```python
from build123d import *

# Parameters (mm, degrees)
SKETCH_1_W          = 56.5
SKETCH_1_H          = 65.5
EXTRUDE_1_DEPTH     = 1.5
SKETCH_2_W          = 59
SKETCH_2_H          = 68
SKETCH_2_W_2        = 56.5
SKETCH_2_H_2        = 65.5
EXTRUDE_2_DEPTH     = 3
FILLET_1_R          = 0.3
SKETCH_4_W          = 25
SKETCH_4_H          = 5
SKETCH_4_W_2        = 30.699386717
SKETCH_4_H_2        = 8.5
SKETCH_4_W_3        = 20
SKETCH_4_H_3        = 30
CUT_EXTRUDE_1_DEPTH = 1
SKETCH_5_W          = 17.035074377
SKETCH_5_H          = 1.25
CUT_EXTRUDE_2_DEPTH = 1.5


with BuildPart() as part:
    # 草图1 → 凸台-拉伸1 (new body)
    with BuildSketch(Plane.XY):
        Rectangle(SKETCH_1_W, SKETCH_1_H)
    extrude(amount=EXTRUDE_1_DEPTH)

    # 草图2 → 凸台-拉伸2 (add)
    with BuildSketch(Plane.XY.offset(1.5)):
        Rectangle(SKETCH_2_W, SKETCH_2_H)
        Rectangle(SKETCH_2_W_2, SKETCH_2_H_2, mode=Mode.SUBTRACT)
    extrude(amount=-EXTRUDE_2_DEPTH)

    # 圆角1
    fillet_1_edges = [part.edges().sort_by_distance(p)[0] for p in [
        (29.5, 34, 0),
        (29.5, -34, 0),
        (-29.5, -34, 0),
        (-29.5, 34, 0),
        (29.5, 0, 1.5),
        (0, 34, 1.5),
        (-29.5, 0, 1.5),
        (0, -34, 1.5),
    ]]
    fillet(fillet_1_edges, radius=FILLET_1_R)

    # 草图4 → 切除-拉伸1 (cut)
    with BuildSketch(Plane(origin=(0, 0, 0), x_dir=(-1, 0, 0), z_dir=(0, 0, -1))):
        with Locations((7.75, 13.75)):
            Rectangle(SKETCH_4_W, SKETCH_4_H)
        with Locations((5.900306641, 5.5)):
            Rectangle(SKETCH_4_W_2, SKETCH_4_H_2)
        with Locations((11.25, -15.75)):
            Rectangle(SKETCH_4_W_3, SKETCH_4_H_3)
    extrude(amount=-CUT_EXTRUDE_1_DEPTH, mode=Mode.SUBTRACT)

    # 草图5 → 切除-拉伸2 (cut)
    with BuildSketch(Plane(origin=(0, 0, -1.5), x_dir=(-1, 0, 0), z_dir=(0, 0, -1))):
        with Locations((-15.836199448, 33.375)):
            Rectangle(SKETCH_5_W, SKETCH_5_H)
    extrude(amount=-CUT_EXTRUDE_2_DEPTH, mode=Mode.SUBTRACT)


solid = part.part
```
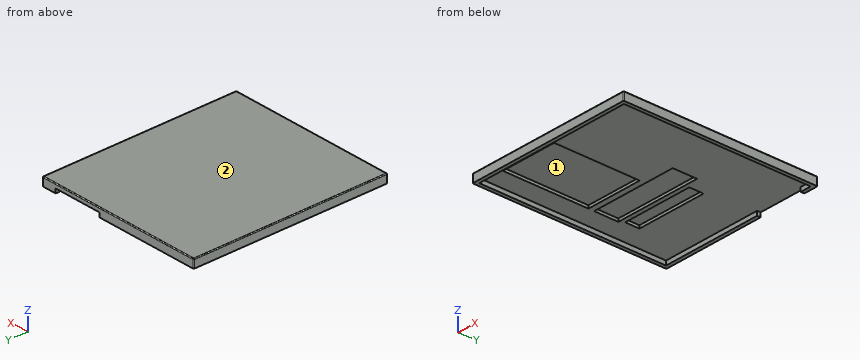
Design review of the part built by this model. Coordinates are the model's own, in mm. Face numbers are marked on the shaded views. Give positions to 0.01 mm unless a question says otherwise; leave off trailing zeros. Loops run counter-clockwise (first coordinate to the right, second up) from the corner with the lowest first, then second, coordinate; pieces in that order, holes last. Notation, with made-up numbers: (67, 8) -> (93, 8) arc R10 ccw to (93, 21) -> close; hole circle Ø4 at (59, 41.5). An arc over 180 degrees is marked (long way). One line per item, written item: value.
Q1. We need section C-C on z = -0.95. Give the boundary of the cut face in (x, y), and give its area (3 significant figures).
Numbers:
outline: (-29.5, -33.7) arc R0.3 ccw to (-29.2, -34) -> (29.2, -34) arc R0.3 ccw to (29.5, -33.7) -> (29.5, 33.7) arc R0.3 ccw to (29.2, 34) -> (24.35, 34) -> (24.35, 32.75) -> (28.25, 32.75) -> (28.25, -32.75) -> (-28.25, -32.75) -> (-28.25, 32.75) -> (7.32, 32.75) -> (7.32, 34) -> (-29.2, 34) arc R0.3 ccw to (-29.5, 33.7) -> close
area: 290 mm^2
Q2. For pin 1 Ø6 at (x, y) = (-5, 12.5) entering from -Z; pin 2 Ø4 at (x, y) = (-7, 7.5) entering from -Z, all flat-tipped, find the tip position at first contact; note any pin that passes through.
Numbers:
pin 1: stops at z = 0
pin 2: stops at z = 1
Q3. We need section B-B on y = 17. Give the boundary of the cut face in (x, z), and give its area (3 significant figures).
Numbers:
outline: (-29.5, -1.5) -> (-28.25, -1.5) -> (-28.25, 0) -> (28.25, 0) -> (28.25, -1.5) -> (29.5, -1.5) -> (29.5, 1.2) arc R0.3 ccw to (29.2, 1.5) -> (-29.2, 1.5) arc R0.3 ccw to (-29.5, 1.2) -> close
area: 92.2 mm^2
Q4. Draft analysis for pull direction Y (two halves, no side actions). For the marked faces 1 and 2, state which applies: pulls with the +Y half, pulls with the -Y half, needs draft (parallel to the pull), parting line crosses it, or undercut.
Numbers:
face 1: undercut
face 2: needs draft
Q5. For L1, parallel to Y at x = -7.5, z = 0.4; L2, parallel to X at y = 7, z = -0.45; L3, parallel to Y at x = 8.5, z = 0.2, list the stretches that pass through material, from the lowest coordinate up.
Numbers:
L1: y = -34 to -30.75, -0.75 to 1.25, 9.75 to 11.25, 16.25 to 34
L2: x = -29.5 to -28.25, 28.25 to 29.5
L3: y = -34 to 1.25, 9.75 to 34
Q6. We need section A-A on x = 22.5. Give the boundary of the cut face in (y, z).
Numbers:
outline: (-34, -1.5) -> (-32.75, -1.5) -> (-32.75, 0) -> (34, 0) -> (34, 1.2) arc R0.3 ccw to (33.7, 1.5) -> (-33.7, 1.5) arc R0.3 ccw to (-34, 1.2) -> close
Q7. We need section D-D on y = 9. Give the boundary of the cut face in (x, z), and give its area (3 significant figures).
Numbers:
outline: (-29.5, -1.5) -> (-28.25, -1.5) -> (-28.25, 0) -> (-21.25, 0) -> (-21.25, 1) -> (9.45, 1) -> (9.45, 0) -> (28.25, 0) -> (28.25, -1.5) -> (29.5, -1.5) -> (29.5, 1.2) arc R0.3 ccw to (29.2, 1.5) -> (-29.2, 1.5) arc R0.3 ccw to (-29.5, 1.2) -> close
area: 61.5 mm^2
